Read the model definition and answer for the solid it produces. Units are mm, in the model's axes. Face numbers are marked on the shaded views. Give positions to 0.01 mm unless a question says otherwise; leave off trailing zeros. Order: outer loops, then holes, each group sorted by start corner. A loop starts at its lowest first (then second) coordinate and runs counter-clockwise, first axis right, second up. Notation, with made-up numbers: M -35,70.5 L 21,70.5 A9 cw 21,77.5 Z; hole C 44,-35.75 d6. An arc over 180 degrees is marked long. Write item = value, one per line. Start each with the question number.
from build123d import *

# Parameters (mm, degrees)
BASE_EXTRUSION_DEPTH    = 9.6
ESQUISSE2_R             = 5
ENL_V_MAT_EXTRU_1_DEPTH = 10.6
ESQUISSE4_R             = 2
ENL_V_MAT_EXTRU_2_DEPTH = 20.2


with BuildPart() as part:
    # Esquisse1 → Base-Extrusion (new body)
    with BuildSketch(Plane.XY):
        Polygon((-11.085125168, 0), (-5.542562584, 9.6), (5.542562584, 9.6), (11.085125168, 0), (5.542562584, -9.6), (-5.542562584, -9.6), align=None)
    extrude(amount=BASE_EXTRUSION_DEPTH)

    # Esquisse2 → Enl_v. mat.-Extru.1 (cut, through all)
    with BuildSketch(Plane.XY.offset(9.6)):
        Circle(ESQUISSE2_R)
    extrude(amount=-ENL_V_MAT_EXTRU_1_DEPTH, mode=Mode.SUBTRACT)

    # Esquisse4 → Enl_v. mat.-Extru.2 (cut, through all)
    with BuildSketch(Plane(origin=(0, 9.6, 0), x_dir=(-1, 0, 0), z_dir=(0, 1, 0))):
        with Locations((0, 4.956948818)):
            Circle(ESQUISSE4_R)
    extrude(amount=-ENL_V_MAT_EXTRU_2_DEPTH, mode=Mode.SUBTRACT)

    # Esquisse6 → Enl_vement de mati_re-R_volution2 (revolve, cut)
    with BuildSketch(Plane(origin=(0, 0, 0), x_dir=(1, 0, 0), z_dir=(0, 1, 0))):
        Polygon((-11.085125168, 0), (-9.595561474, 0), (-11.085125168, -0.86), align=None)
        Polygon((-11.085125168, -8.74), (-11.085125168, -9.6), (-9.595561474, -9.6), align=None)
    revolve(axis=Axis((0, 0, 0), (0, 0, 1)), mode=Mode.SUBTRACT)


solid = part.part
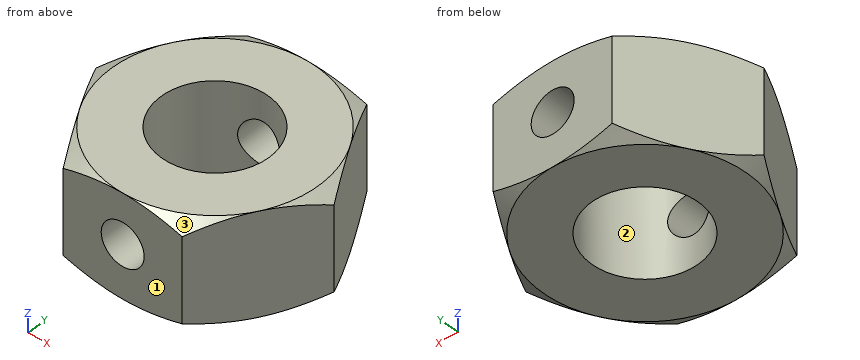
1) For a pull along X with two mould halves and no side action, classify the marked faces 1, 2 and 3 as pulls with the +X half, pulls with the -X half, needs draft (parallel to the pull), parting line crosses it, or undercut.
2) Find section B-B on z = 2.25. Determine the outline of the cut face in (x, y), plus the area to 3 significant figures.
3) Each of these flat-tipped pins is pushed along its axis until it touches: P1, Ø5, axis at y = -5.5, z = 3.5, coming from the -X side; P2, Ø2, axis at y = -5, z = 5, coming from the -X side. Where does it stop, or does it pass through?
4) Find section C-C on z = 6.5. Determine the outline of the cut face in (x, y).
5) Find the intervals of material crossed by probe 1 along Z at (x, y) = (0, -8); probe 2 along X at (y, z) = (-0.5, 5); probe 3 along X at (y, z) = (-1.5, 6.25), in increasing order. Write a range as [from, to].
6) Find section A-A on x = 0. Count the separate pieces of the cut face and the enclosed holes in it, plus the area to 3 significant figures.
Numbers:
q1.face_1 = needs draft
q1.face_2 = undercut
q1.face_3 = parting line crosses it
q2.outline = M -11.09,0 L -5.54,-9.6 L 5.54,-9.6 L 11.09,0 L 5.54,9.6 L -5.54,9.6 Z; hole C 0,0 d10
q2.area = 241 mm2
q3.P1 = -9.35
q3.P2 = -8.78
q4.outline = M -11.09,0 L -5.54,-9.6 L -1.27,-9.6 L -1.27,-4.84 A5 cw -1.27,4.84 L -1.27,9.6 L -5.54,9.6 Z; M 1.27,-9.6 L 5.54,-9.6 L 11.09,0 L 5.54,9.6 L 1.27,9.6 L 1.27,4.84 A5 cw 1.27,-4.84 Z
q5.probe_1 = [0, 2.96], [6.96, 9.6]
q5.probe_2 = [-10.8, -4.97], [4.97, 10.8]
q5.probe_3 = [-10.22, -4.77], [4.77, 10.22]
q6.separate_pieces = 4
q6.enclosed_holes = 0
q6.area = 51.5 mm2
